Design review of the part built by this model. Coordinates are the model's own, in mm. Face numbers are marked on the shaded views. A direction names the side the tool comes from. Coordinates: 2 decimals unless noted, no trailing zeros. Write each loop counter-clockwise with the first axis right and the second up, starting at its lowest first coordinate (ties: lowest second). Pieces come first, ordered by that corner, then holes. Notation, with made-up numbers: (12, 87) - (28, 87) arc R12 cw to (28, 99) - close; hole circle Ø4 at (-19.75, 10). An arc over 180 degrees is marked (long way). Use a Markdown table: item, result.
from build123d import *

# Parameters (mm, degrees)
SKETCH1_R           = 54.929
SKETCH1_R_2         = 11.176
BOSS_EXTRUDE1_DEPTH = 6.985
CUT_EXTRUDE1_DEPTH  = 6.985


with BuildPart() as part:
    # Sketch1 → Boss-Extrude1 (new body)
    with BuildSketch(Plane.XY):
        with Locations((-9.1425, 0)):
            Circle(SKETCH1_R)
        with Locations((-9.1425, 0)):
            Circle(SKETCH1_R_2, mode=Mode.SUBTRACT)
    extrude(amount=BOSS_EXTRUDE1_DEPTH)

    # Sketch2 → Cut-Extrude1 (cut)
    with BuildSketch(Plane.XY.offset(6.985)):
        Polygon((35.7865, -17.654216531), (5.2085, 0), (35.7865, 17.654216531), align=None)
        Polygon((5.067651025, -46.134130643), (-0.194797854, -11.220063605), (32.67289559, -24.119682709), align=None)
        Polygon((-36.351731506, -39.874103416), (-12.335897923, -13.991190468), (-1.928554578, -47.730968917), align=None)
        Polygon((-57.282007746, -3.588063033), (-22.072304223, -6.22666554), (-41.962252786, -35.399861997), align=None)
        Polygon((-41.962252786, 35.399861997), (-22.072304223, 6.22666554), (-57.282007746, 3.588063033), align=None)
        Polygon((-1.928554578, 47.730968917), (-12.335897923, 13.991190468), (-36.351731506, 39.874103416), align=None)
        Polygon((32.67289559, 24.119682709), (-0.194797854, 11.220063605), (5.067651025, 46.134130643), align=None)
    extrude(amount=-CUT_EXTRUDE1_DEPTH, mode=Mode.SUBTRACT)


solid = part.part
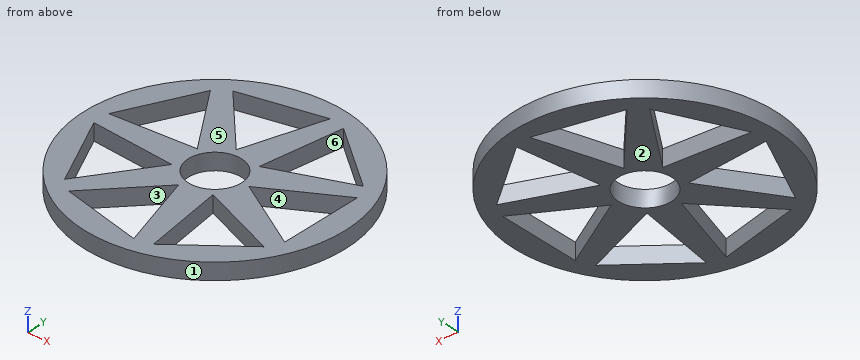
(1) Take a section at D-D on x = -54.5. Write out the cut boundary in (y, z) (3 decimals).
Determined:
| item | result |
|---|---|
| outline | (-30.982, 0) - (-9.365, 0) - (-9.365, 6.985) - (-30.982, 6.985) - close; (-3.797, 0) - (3.797, 0) - (3.797, 6.985) - (-3.797, 6.985) - close; (9.365, 0) - (30.982, 0) - (30.982, 6.985) - (9.365, 6.985) - close |
(2) Draft analysis for pull direction Y (two halves, no side actions). For the marked faces 1, 2, 3 and 4, state which applies: +Y half, -Y half, draft (parallel to the pull), parting line (faces both ways), or undercut.
Determined:
| item | result |
|---|---|
| face 1 | parting line |
| face 2 | draft |
| face 3 | undercut |
| face 4 | undercut |
(3) Take a section at B-B on x = 16. Write out the cut boundary in (y, z) (3 decimals).
Determined:
| item | result |
|---|---|
| outline | (-48.837, 0) - (-37.416, 0) - (-37.416, 6.985) - (-48.837, 6.985) - close; (-17.576, 0) - (-6.23, 0) - (-6.23, 6.985) - (-17.576, 6.985) - close; (6.23, 0) - (17.576, 0) - (17.576, 6.985) - (6.23, 6.985) - close; (37.416, 0) - (48.837, 0) - (48.837, 6.985) - (37.416, 6.985) - close |
(4) For L1, parallel to Y at x = -25, z = 1; L2, parallel to Y at x = -52, z = 3.5; L3, parallel to X at y = 33.5, z = 2.25, list the stretches that pass through material, from the lowest coordinate up. Write a range as from..to.
Determined:
| item | result |
|---|---|
| L1 | -52.59..-42.47, -27.64..-10.52, -6.01..6.01, 10.52..27.64, 42.47..52.59 |
| L2 | -34.36..-14.56, -3.98..3.98, 14.56..34.36 |
| L3 | -52.67..-42.88, -40.67..-30.44, -6.32..3.16, 20.91..34.39 |
(5) For pin 1 (18 mm diameter, centred on x = -9.14, y = 0, fed in from +Z); pin 2 (1.5 mm diameter, centred on x = 7, z = 3.5, fed in from -Y); pin 3 (2 mm diameter, centred on y = 4.5, z = 3.5, fed in from -X); pin 4 (3 mm diameter, centred on y = 13.5, z = 4, fed in from +X), all flat-tipped, find the tip position at first contact; note any pin that passes through.
Determined:
| item | result |
|---|---|
| pin 1 | through |
| pin 2 | y = -52.73 |
| pin 3 | x = -63.96 |
| pin 4 | x = 44.46 |
(6) Take a section at C-C on z = 2. State how many separate pieces and enclosed holes the cut face has, and give its area (3 significant figures).
Determined:
| item | result |
|---|---|
| separate pieces | 1 |
| enclosed holes | 8 |
| area | 5,310 mm2 |
(7) Machinability: for the marked faces 5 and 6, which of the approach directions +Z, -Z, +X, -X, +Y, -Y give a long, thin tool a straight path to every point of the face, cutting with its end or side? Answer none if there is none.
Determined:
| item | result |
|---|---|
| face 5 | +Z, +X, -X, +Y, -Y |
| face 6 | +Z, -Z |
(8) Take a section at A-A on y = 8. Write out the cut boundary in (x, z) (1 decimal).
Determined:
| item | result |
|---|---|
| outline | (-63.5, 0) - (-55.2, 0) - (-55.2, 7) - (-63.5, 7) - close; (-23.3, 0) - (-16.9, 0) - (-16.9, 7) - (-23.3, 7) - close; (-1.3, 0) - (19.1, 0) - (19.1, 7) - (-1.3, 7) - close; (35.8, 0) - (45.2, 0) - (45.2, 7) - (35.8, 7) - close |
